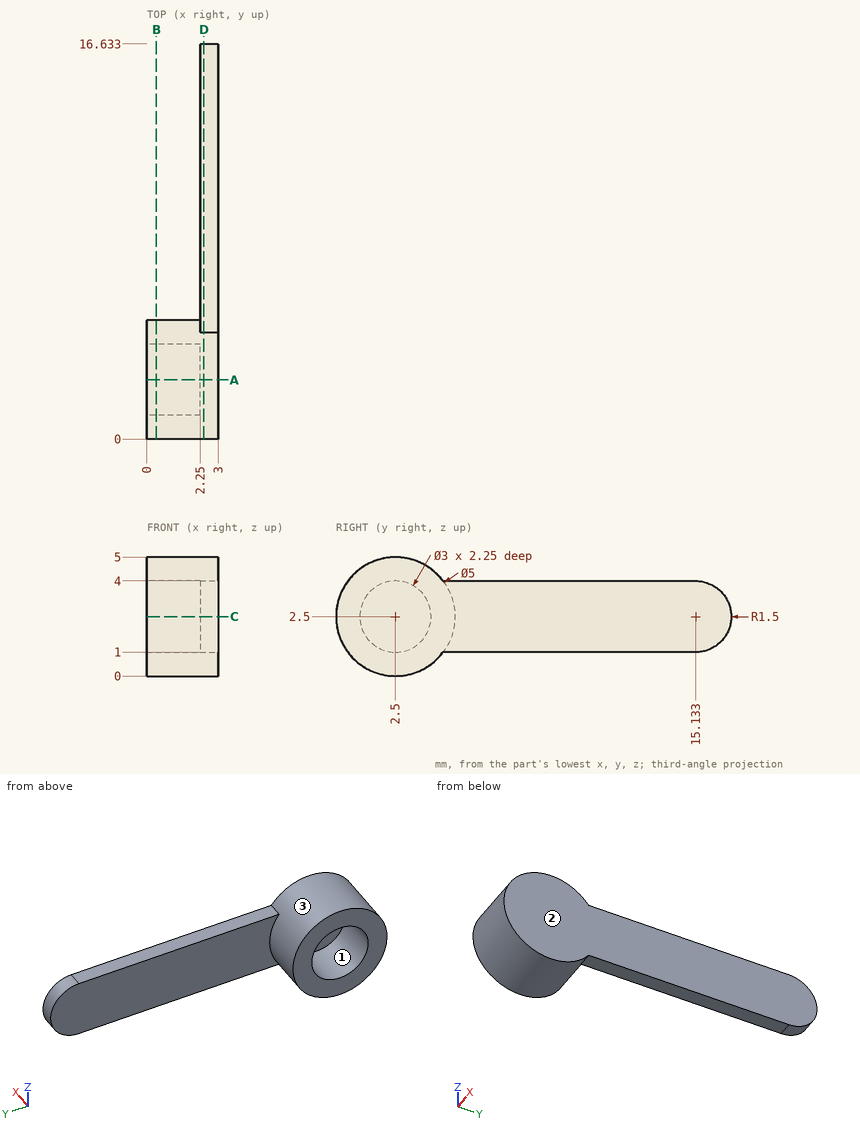
Answer from the drawing. Dimensions are ordinates in mm from the lowest x, y and z of the part. Coordinates: 2 decimals unless noted, no trailing zeros. Write each loop counter-clockwise with the first axis right and the second up, starting at its lowest first coordinate (ties: lowest second). Pieces come first, ordered by that corner, then holes. Notation, with made-up numbers: (-20, 49.5) - (-16, 49.5) arc R20 ccw to (-16, 78.5) - close; hole circle Ø3 at (-11, 11). An arc over 180 degrees is marked (long way). One line per question, with ' | ' between items.
Q1. Each of these flat-tipped pins is pushed along its axis until it touches: P1, Ø1.5, axis at x = 2, y = 12.5, coming from the -Z side; P2, Ø0.9, axis at y = 2.5, z = 2, coming from the -X side; P3, Ø0.6, axis at x = 3, y = 11.5, coming from the +Z side. Where does it stop, or does it pass through?
Result set:
P1: z = 1 | P2: x = 2.25 | P3: z = 4
Q2. Consider L1, parallel to Y at x = 1.15, z = 2.5; L2, parallel to X at y = 12.5, z = 3.8. Determine where each line is inside the solid, lowest interval first. Write a range as [from, to].
Result set:
L1: [0, 1], [4, 5] | L2: [2.25, 3]
Q3. Find section D-D, the plane x = 2.4. Write down the section's boundary in (y, z).
Result set:
outline: (4.5, 1) - (15.13, 1) arc R1.5 ccw to (15.13, 4) - (4.5, 4) arc R2.5 ccw (long way) to start
Q4. Find section C-C, the plane z = 2.5. Write down the section's boundary in (x, y), plus the area to 3 significant figures.
Result set:
outline: (0, 0) - (3, 0) - (3, 16.63) - (2.25, 16.63) - (2.25, 5) - (0, 5) - (0, 4) - (2.25, 4) - (2.25, 1) - (0, 1) - close | area: 17.0 mm^2
Q5. Determine the mould class of the marked faces 1, 2 and 3 for opening direction Y: +Y half, -Y half, draft (parallel to the pull), parting line (faces both ways), or undercut.
Result set:
face 1: undercut | face 2: draft | face 3: parting line
Q6. Find section B-B, the plane x = 0.4. Write down the section's boundary in (y, z).
Result set:
outline: circle Ø5 at (2.5, 2.5); hole circle Ø3 at (2.5, 2.5)
Q7. Find section A-A, the plane y = 2.5. Write down the section's boundary in (x, z).
Result set:
outline: (0, 0) - (3, 0) - (3, 5) - (0, 5) - (0, 4) - (2.25, 4) - (2.25, 1) - (0, 1) - close
